For this review, use the dimensioned drawing (mm, ordinates from the lowest corner) and the shaded views. A direction names the side the tool comes from. Coordinates: 2 decimals unless noted, no trailing zeros. Order: outer loops, then holes, each group sorted by start corner. A loop starts at its lowest first (then second) coordinate and runs counter-clockwise, first axis right, second up. Notation, with made-up numbers: M 52,20.25 L 105,20.25 A9 cw 105,34.25 Z; hole C 8.25,32 d5. An arc over 180 degrees is marked long. Answer in a Markdown table with one row per item.
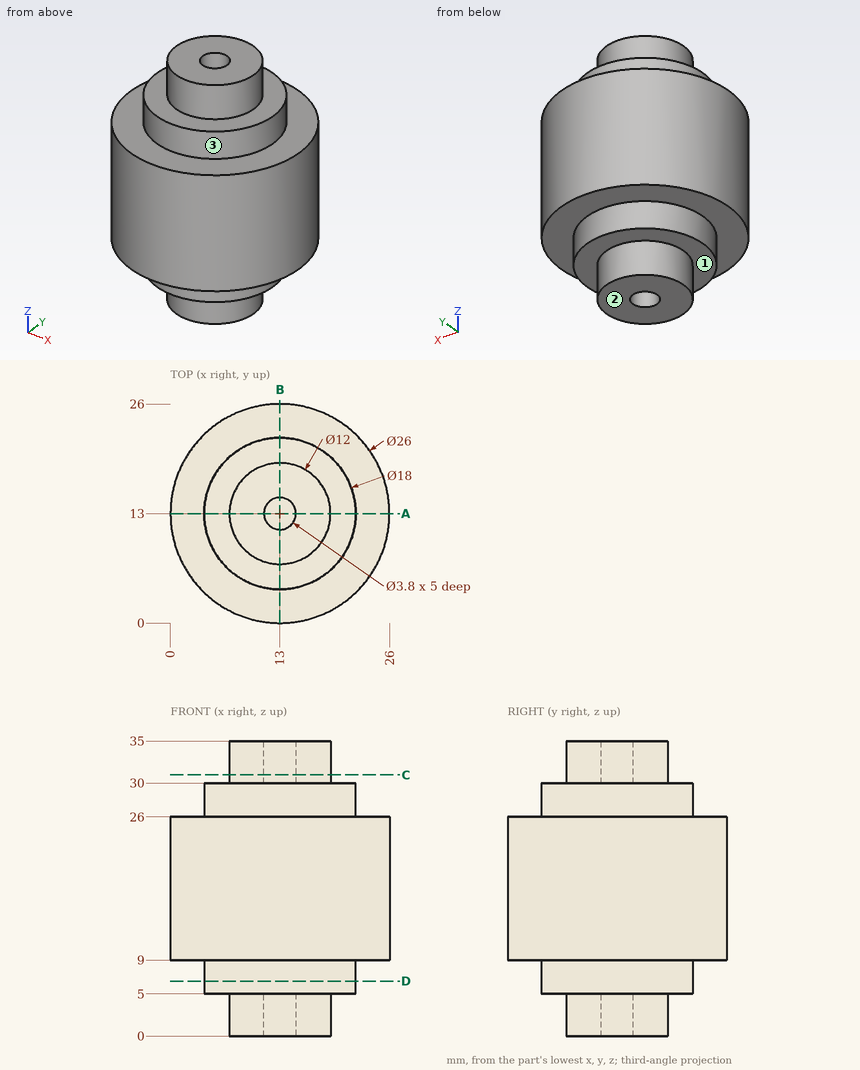
(1) Take a section at C-C (z = 31). Write out the cut boundary in (x, y), then the cut area to 3 significant figures.
Report:
| item | result |
|---|---|
| outline | C 13,13 d12; hole C 13,13 d3.8 |
| area | 102 mm^2 |
(2) To check wall thickness, follow line 1 (Y direction, x = 13, z = 2.95); line 2 (Z direction, x = 6.75, y = 14.25); line 3 (X direction, y = 12.75, z = 24.5). State the ranges of each line that lie inside material, in increasing order. Write a range as [from, to].
Report:
| item | result |
|---|---|
| line 1 | [7, 11.1], [14.9, 19] |
| line 2 | [5, 30] |
| line 3 | [0, 26] |
(3) Insertion check: P1, Ø1.1, axis at x = 12.5, y = 13.5, coming from the +Z side; P2, Ø1.5, axis at y = 6, z = 5, coming from the -X side; P3, Ø1.5, axis at x = 16.5, z = 23, coming from the -Y side. Each pin has a flat end and moves straight along its axis. Give the tip position at first contact, or say it passes through.
Report:
| item | result |
|---|---|
| P1 | z = 30 |
| P2 | x = 6.52 |
| P3 | y = 0.29 |
(4) Take a section at D-D (z = 6.5). Write out the cut boundary in (x, y), then the cut area to 3 significant figures.
Report:
| item | result |
|---|---|
| outline | C 13,13 d18 |
| area | 254 mm^2 |
(5) Machinability: for the marked faces 1, 2 and 3, which of the approach directions +Z, -Z, +X, -X, +Y, -Y give a long, thin tool a straight path to every point of the face, cutting with its end or side? Answer none if there is none.
Report:
| item | result |
|---|---|
| face 1 | -Z |
| face 2 | -Z, +X, -X, +Y, -Y |
| face 3 | +Z |
(6) Take a section at A-A (y = 13). Write out the cut boundary in (x, z), then the cut area to 3 significant figures.
Report:
| item | result |
|---|---|
| outline | M 0,9 L 4,9 L 4,5 L 7,5 L 7,0 L 11.1,0 L 11.1,5 L 14.9,5 L 14.9,0 L 19,0 L 19,5 L 22,5 L 22,9 L 26,9 L 26,26 L 22,26 L 22,30 L 19,30 L 19,35 L 14.9,35 L 14.9,30 L 11.1,30 L 11.1,35 L 7,35 L 7,30 L 4,30 L 4,26 L 0,26 Z |
| area | 668 mm^2 |
